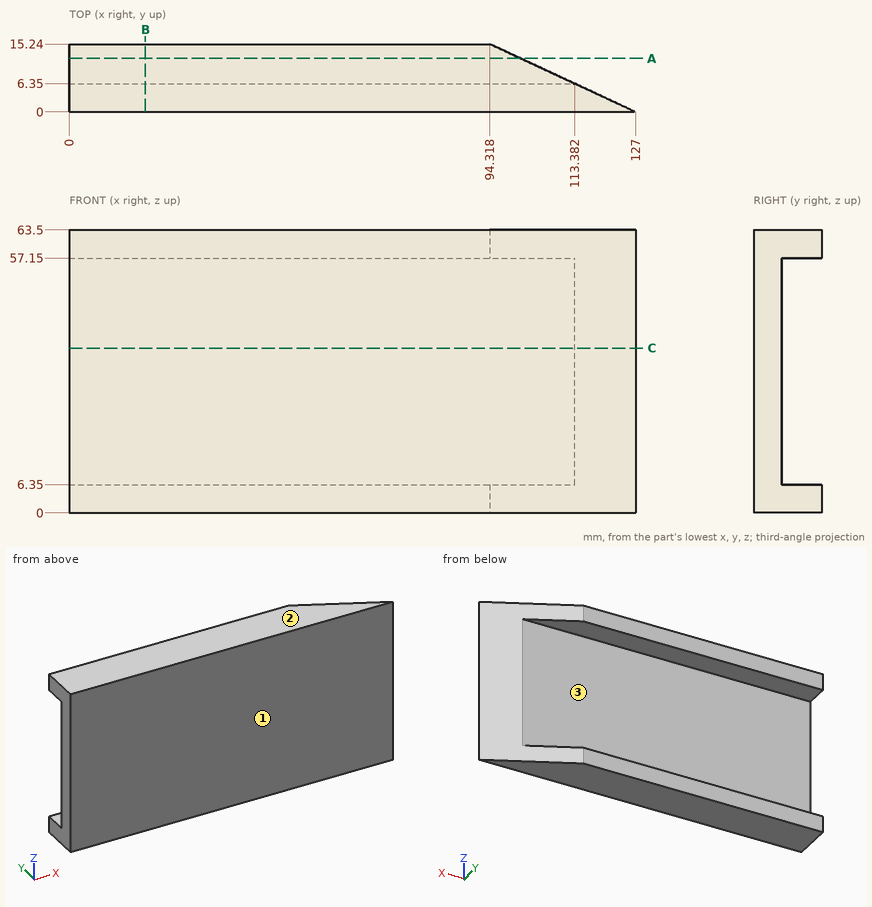
Here's the drawing with two shaded views (mm, measured from the low corner). I have some questions. Coordinates: 2 decimals unless noted, no trailing zeros. Write each loop counter-clockwise with the first axis right and the second up, starting at its lowest first coordinate (ties: lowest second). Pieces come first, ordered by that corner, then holes.
Item 1: I want a section at C-C on z = 37. Write out the boundary of the cut face in (x, y).
Item 2: I want a section at A-A on y = 12. Write out the boundary of the cut face in (x, z), and give its area (3 significant figures).
Item 3: If I drill on line 1 (Z direction, x = 63, y = 7); line 2 (Y direction, x = 36, z = 37); line 3 (X direction, y = 5.75, z = 15.5), over which ranges is the centre line in solid material (lowest first)?
Item 4: I want a section at B-B on x = 17. Write out the boundary of the cut face in (y, z).
Item 5: If we mould it in two halves opening along Z, with no side actions, what happens to the marked faces 1, 2 and 3? For each: +Z half, -Z half, draft (parallel to the pull), parting line (faces both ways), or undercut.
Item 6: Will these pins go through, and if not, where does the flat tip stop? pin 1 (12 mm diameter, centred on x = 26, z = 24, fed in from +Y); pin 2 (1 mm diameter, centred on y = 7, z = 53.5, fed in from +X).
Findings below:
1. outline: (0, 0) - (127, 0) - (113.38, 6.35) - (0, 6.35) - close
2. outline: (0, 0) - (101.27, 0) - (101.27, 6.35) - (0, 6.35) - close; (0, 57.15) - (101.27, 57.15) - (101.27, 63.5) - (0, 63.5) - close
2. area: 1,290 mm2
3. line 1: z = 0 to 6.35, 57.15 to 63.5
3. line 2: y = 0 to 6.35
3. line 3: x = 0 to 114.67
4. outline: (0, 0) - (15.24, 0) - (15.24, 6.35) - (6.35, 6.35) - (6.35, 57.15) - (15.24, 57.15) - (15.24, 63.5) - (0, 63.5) - close
5. face 1: draft
5. face 2: +Z half
5. face 3: undercut
6. pin 1: stops at y = 6.35
6. pin 2: passes through
